CAD build for the part. Positions are in the model's coordinates, mm. A direction names the side the tool comes from. Give positions to 0.01 mm unless a question says otherwise; leave off trailing zeros. Loops run counter-clockwise (first coordinate to the right, second up) from the corner with the lowest first, then second, coordinate; pieces in that order, holes last.
```python
from build123d import *

# Parameters (mm, degrees)
F0_R     = 38.903561
F1_DEPTH = 40
F2_DEPTH = 10
F4_DEPTH = 30
F6_DEPTH = 20


with BuildPart() as f1:
    # F0 (on Top) → F1 (new body)
    with BuildSketch(Plane.XY):
        with BuildLine():
            ThreePointArc((145.735341, -0.967313), (122.074479, 43.625472), (71.883693, 49.032687))
            ThreePointArc((71.883693, 49.032687), (38.032045, -0.967313), (71.883693, -50.967313))
            ThreePointArc((71.883693, -50.967313), (122.074479, -45.560098), (145.735341, -0.967313))
        make_face()
        with Locations((91.883693, -0.967313)):
            Circle(F0_R, mode=Mode.SUBTRACT)
    extrude(amount=F1_DEPTH)

    # F0 (on Top) → F2 (join)
    with BuildSketch(Plane.XY):
        with BuildLine():
            Line((71.883693, 49.032687), (-44.412829, 49.032687))
            Line((-44.412829, 49.032687), (-44.412829, -50.967313))
            Line((-44.412829, -50.967313), (71.883693, -50.967313))
            ThreePointArc((71.883693, -50.967313), (38.032045, -0.967313), (71.883693, 49.032687))
        make_face()
    extrude(amount=F2_DEPTH)

    # F3 (on face) → F4 (join)
    with BuildSketch(Plane.XY.offset(10)):
        with BuildLine():
            ThreePointArc((38.968667, -10.967313), (38.032045, -0.967313), (38.968667, 9.032687))
            Line((38.968667, 9.032687), (-24.967955, 9.032687))
            Line((-24.967955, 9.032687), (-24.967955, -0.967313))
            Line((-24.967955, -0.967313), (-24.967955, -10.967313))
            Line((-24.967955, -10.967313), (38.968667, -10.967313))
        make_face()
    extrude(amount=F4_DEPTH)

    # F5 (on face) → F6 (cut)
    with BuildSketch(Plane.XZ.offset(10.967313)):
        Polygon((-24.967955, 40), (-24.967955, 10), (38.968667, 40), align=None)
    extrude(amount=-F6_DEPTH, mode=Mode.SUBTRACT)


solid = f1.part
```
1. Saw through at A-A, the plane x = 57.5. List the corners of the cut face in (y, z).
Responses:
outline: (-50.97, 0) - (-19.17, 0) - (-19.17, 40) - (-42.41, 40) - (-42.41, 10) - (-50.97, 10) - close; (17.23, 0) - (49.03, 0) - (49.03, 10) - (40.48, 10) - (40.48, 40) - (17.23, 40) - close
2. Saw through at B-B, the plane y = -14.5. List the corners of the cut face in (x, z), and give its area (3 significant figures).
Responses:
outline: (-44.41, 0) - (55.41, 0) - (55.41, 40) - (39.76, 40) - (39.76, 10) - (-44.41, 10) - close; (128.36, 0) - (144.01, 0) - (144.01, 40) - (128.36, 40) - close
area: 2,090 mm2
3. Saw through at D-D, the plane x = 35.5. List the corners of the cut face in (y, z).
Responses:
outline: (-50.97, 0) - (49.03, 0) - (49.03, 10) - (9.03, 10) - (9.03, 38.37) - (-10.97, 38.37) - (-10.97, 10) - (-50.97, 10) - close
4. Probe line 1 along Y through (x, z) = (12, 16); line 2 along Z through (x, y) = (-23, -25); line 3 along X through (y, z) = (-5, 28). List the from-to ranges inside material, lowest first.
Responses:
line 1: y = -10.97 to 9.03
line 2: z = 0 to 10
line 3: x = 13.39 to 53.19, 130.58 to 145.58
5. Pull direction X, two halves, no side cores. Call faces 6 (the face through (-44.413, 0, 5)), 7 (the face through (28, 0, 0)), 8 (the face through (53.018, 0.743, 19.72)): released by +X, released by -X, zero draft, split by the parting line, or undercut.
Responses:
face 6: released by -X
face 7: zero draft
face 8: undercut
6. Tool access for faces 1 (the face through (13, -50.967, 5)), 2 (the face through (15, 9.033, 21)), 3 (the face through (0, 11, 10)), 4 (the face through (15, 49.033, 5)), 5 (the face through (21, -10.967, 18)): list every direction of +Z, -Z, +X, -X, +Y, -Y with a clear straight run to the whole face (end or side of a thin tool).
Responses:
face 1: +Z, -Z, -X, -Y
face 2: +Z, -X, +Y
face 3: +Z, -X
face 4: +Z, -Z, -X, +Y
face 5: +Z, -X, -Y
7. Saw through at C-C, the plane z = 22.5. List the corners of the cut face in (x, y).
Responses:
outline: (1.67, -10.97) - (38.97, -10.97) arc R53.85 ccw (long way) to (38.97, 9.03) - (1.67, 9.03) - close; hole circle Ø77.81 at (91.88, -0.97)
8. Drop flat-ended pins along their axis: pin 1 (3 mm diameter, centred on x = 0.5, z = 3.5, fed in from -Y); pin 2 (5 mm diameter, centred on y = -7.5, z = 34, fed in from +X); pin 3 (9 mm diameter, centred on x = 12, z = 18, fed in from -Y). Give the stop position or say it passes through.
Responses:
pin 1: stops at y = -50.97
pin 2: stops at x = 145.58
pin 3: stops at y = -10.97
